Source: three-view drawing plus pictorial views. Frame: mm from the lowest corner of the part. A direction names the side the tool comes from. Coordinates: 2 decimals unless noted, no trailing zeros. Order: outer loops, then holes, each group sorted by start corner. A loop starts at its lowest first (then second) coordinate and runs counter-clockwise, first axis right, second up. Notation, with made-up numbers: (-22.75, -3.5) -> (24.25, -3.5) arc R27 cw to (24.25, 17.5) -> close; hole circle Ø2 at (2, 6). An arc over 180 degrees is marked (long way). One line per question, with ' | ' between items.
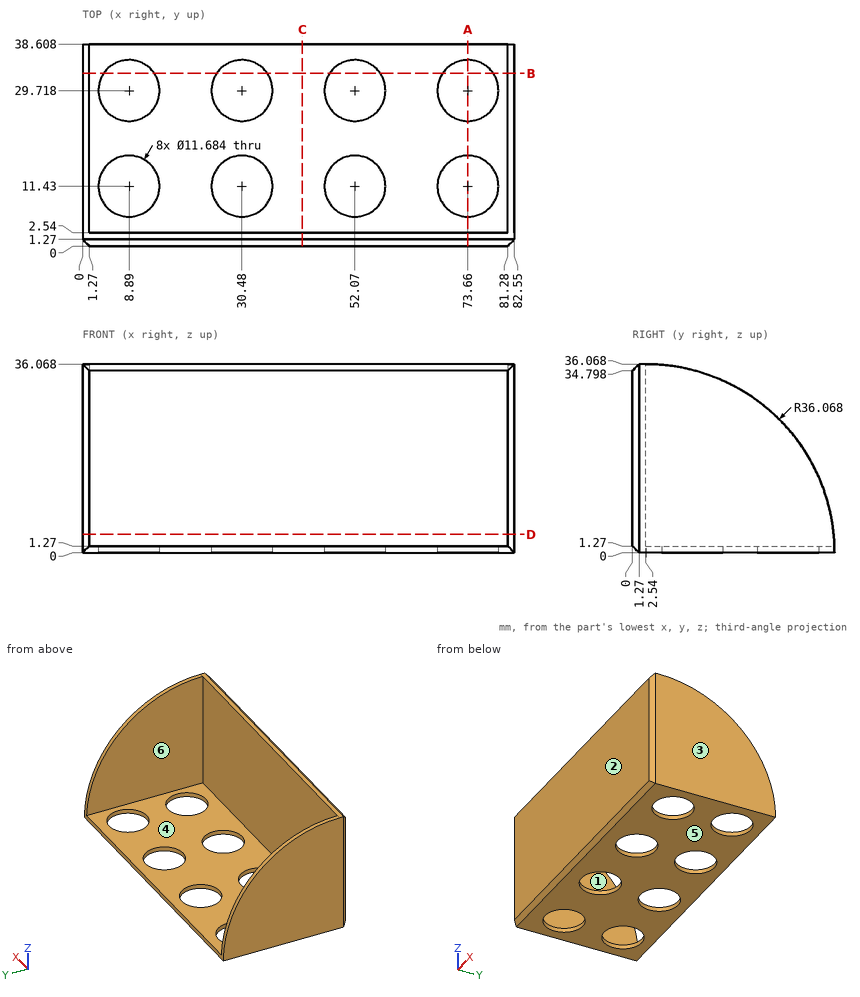
1. Cut plane D-D, the plane z = 3.5. Return loops of the section in (x, y).
Recorded:
outline: (0, 1.27) -> (1.27, 0) -> (81.28, 0) -> (82.55, 1.27) -> (82.55, 38.44) -> (81.28, 38.44) -> (81.28, 2.54) -> (1.27, 2.54) -> (1.27, 38.44) -> (0, 38.44) -> close
2. Access query for the marked faces 1 and 2. Directions: +Z, -Z, +X, -X, +Y, -Y. A direction counts if a zero-diameter tool reaches every point of the face in a straight line with its end or side. Return the directions, or none.
Recorded:
face 1: +Z, +Y | face 2: +Z, -Z, +X, -X, -Y
3. Pin query (flat end, axial travel): pin 1 Ø2 at (x, y) = (71.5, 24.5) entering from +Z; pin 2 Ø8 at (x, z) = (9, 12.5) entering from +Y. Return the tip coordinate at first contact, or that it passes through.
Recorded:
pin 1: stops at z = 1.27 | pin 2: stops at y = 2.54
4. Cut plane C-C, the plane x = 42. Return loops of the section in (y, z), and give its area (3 significant figures).
Recorded:
outline: (0, 1.27) -> (1.27, 0) -> (38.61, 0) arc R36.07 ccw to (38.59, 1.27) -> (2.54, 1.27) -> (2.54, 36.07) -> (1.27, 36.07) -> (0, 34.8) -> close | area: 136 mm^2
5. Mould query, pull axis X, two halves, no side actions, for the marked faces 3, 4, 5 and 6. Classes: released by +X, released by -X, zero draft, split by the parting line, or undercut.
Recorded:
face 3: released by +X | face 4: undercut | face 5: zero draft | face 6: undercut
6. Cut plane A-A, the plane x = 73.66. Return loops of the section in (y, z).
Recorded:
outline: (0, 1.27) -> (1.27, 0) -> (5.59, 0) -> (5.59, 1.27) -> (2.54, 1.27) -> (2.54, 36.07) -> (1.27, 36.07) -> (0, 34.8) -> close; (17.27, 0) -> (23.88, 0) -> (23.88, 1.27) -> (17.27, 1.27) -> close; (35.56, 0) -> (38.61, 0) arc R36.07 ccw to (38.59, 1.27) -> (35.56, 1.27) -> close
7. Cut plane B-B, the plane y = 33. Return loops of the section in (x, z), and give its area (3 significant figures).
Recorded:
outline: (0, 0) -> (4.06, 0) -> (4.06, 1.27) -> (1.27, 1.27) -> (1.27, 19.32) -> (0, 19.32) -> close; (13.72, 0) -> (25.65, 0) -> (25.65, 1.27) -> (13.72, 1.27) -> close; (35.31, 0) -> (47.24, 0) -> (47.24, 1.27) -> (35.31, 1.27) -> close; (56.9, 0) -> (68.83, 0) -> (68.83, 1.27) -> (56.9, 1.27) -> close; (78.49, 0) -> (82.55, 0) -> (82.55, 19.32) -> (81.28, 19.32) -> (81.28, 1.27) -> (78.49, 1.27) -> close | area: 102 mm^2
8. Ray query, line 1 (X direction, y = 13, z = 22); line 2 (Y direction, x = 30.48, z = 0.4); line 3 (Y direction, x = 78, z = 1). Return the intervals inside material, ascending. Write a range as [from, to].
Recorded:
line 1: x = [0, 1.27], [81.28, 82.55] | line 2: y = [0.87, 5.59], [17.27, 23.88], [35.56, 38.61] | line 3: y = [0.27, 7.52], [15.34, 25.81], [33.63, 38.59]
